Autodesk Inventor part; units mm, degrees
ref_plane "YZ Plane" through (0, 0, 0) normal (1, 0, 0) x (0, 1, 0)
ref_plane "XZ Plane" through (0, 0, 0) normal (0, 1, 0) x (-1, 0, 0)
ref_plane "XY Plane" through (0, 0, 0) normal (0, 0, 1) x (1, 0, 0)
sketch "Sketch1" plane through (0, 0, 0) normal (0, 1, 0) x (-1, 0, 0)
  line L0 (0, 0) -> (20, 0)
  line L1 (20, 0) -> (20, -20)
  line L2 (20, -20) -> (0, -20)
  line L3 (0, -20) -> (0, 0)
  point P0 (0, -10)
  point P1 (20, -10)
  dimension "d0" = 20
  dimension "d1" = 20
extrude "Extrusion1" add sketch "Sketch1" along normal blind 10
sketch "Sketch2" plane through (0, 0, 0) normal (0, -1, 0) x (1, 0, 0)
  circle A0 centre (-10, -10) radius 2.1511
  line L0 (-20, 0) -> (0, 0)
  line L1 (-13.8262, -12.1511) -> (-13.776, -7.7619)
  line L2 (-13.776, -7.7619) -> (-9.9498, -5.6108)
  line L3 (-9.9498, -5.6108) -> (-6.1738, -7.8489)
  line L4 (-6.1738, -7.8489) -> (-6.224, -12.2381)
  line L5 (-6.224, -12.2381) -> (-10.0502, -14.3892)
  line L6 (-10.0502, -14.3892) -> (-13.8262, -12.1511)
  dimension "d4" = 10
extrude "Extrusion2" cut sketch "Sketch2" against normal blind 1 contours A0 | L1 L2 L3 L4 L5 L6
sketch "Sketch3" plane through (0, 1, 0) normal (0, -1, 0) x (1, 0, 0)
  circle A0 centre (-9.9498, -10) radius 3
  line L0 (-20, 0) -> (0, 0)
  point P0 (-10, 0)
  dimension "d7" = 6
  dimension "d8" = 10
extrude "Extrusion3" cut sketch "Sketch3" against normal blind 8.5
sketch "Sketch4" plane through (0, 10, 0) normal (0, 1, 0) x (1, 0, 0)
  line L0 (0, 0) -> (0, 20)
  line L1 (-20, 20) -> (-20, 0)
  line L2 (0, 0) -> (-20, 20)
  line L3 (-20, 20) -> (-20, 0)
  line L4 (-20, 0) -> (0, 20)
  line L5 (0, 20) -> (0, 10)
  line L6 (0, 10) -> (-20, 10)
  line L7 (-20, 0) -> (0, 0)
  line L8 (-10, 0) -> (-10, 20)
  line L9 (-3.5295, 15.6) -> (-10, 15.6)
  line L10 (-10, 15.6) -> (-10, 12.6)
  line L11 (-10, 12.6) -> (-3.5295, 12.6)
  line L12 (-3.5295, 12.6) -> (-3.5295, 15.6)
  line L13 (-16.4705, 15.6) -> (-10, 15.6)
  line L14 (-10, 12.6) -> (-16.4705, 12.6)
  line L15 (-16.4705, 12.6) -> (-16.4705, 15.6)
  line L16 (-3.5295, 4.4) -> (-10, 4.4)
  line L17 (-10, 7.4) -> (-3.5295, 7.4)
  line L18 (-3.5295, 7.4) -> (-3.5295, 4.4)
  line L19 (-10, 7.4) -> (-16.4705, 7.4)
  line L20 (-16.4705, 7.4) -> (-16.4705, 4.4)
  line L21 (-16.4705, 4.4) -> (-10, 4.4)
  point P0 (-6.7648, 12.6)
  point P1 (-6.7648, 15.6)
  dimension "d11" = 3
  dimension "d18" = 5.2
extrude "Extrusion4" add sketch "Sketch4" along normal blind 10 contours L16 L8 L17 L2 | L2 L17 L18 L16 | L21 L4 L19 L8 | L9 L12 L11 L4 | L4 L11 L8 L9 | L14 L15 L13 L2 | L2 L13 L8 L14 | L4 L21 L20 L19
sketch "Sketch5" plane through (-3.5295, 10, -15.6) normal (0, 0, -1) x (-1, 0, 0)
  circle A0 centre (6.4705, 5) radius 2.75
  line L0 (0, 10) -> (12.941, 10)
  line L1 (16.4705, 0) -> (-3.5295, 0)
  line L2 (0, 0) -> (0, 10)
  line L3 (12.941, 0) -> (12.941, 10)
  point P0 (-3.5295, -10)
  dimension "d14" = 5.5
  dimension "d15" = 5
  dimension "d19" = 10
  dimension "d20" = 12.941
extrude "Extrusion5" cut sketch "Sketch5" against normal blind 66.5 contours A0
properties part number "RollZ" material "Thermoplastic Resin"
Geometry check sheet. Reference: the model listing, model coordinates, mm. A direction names the side the tool comes from. Coordinates: 2 decimals unless noted, no trailing zeros. Order: outer loops, then holes, each group sorted by start corner. A loop starts at its lowest first (then second) coordinate and runs counter-clockwise, first axis right, second up. Notation, with made-up numbers: (-19, -25.75) - (31, -25.75) arc R18 ccw to (31, -1.75) - close; hole circle Ø6 at (-21, 45). An arc over 180 degrees is marked (long way). Answer as a JSON object with one key per item and string values. Group by question number.
Item 1: Tool access check on faces 4 (the face through (-3.53, 15, -14)), 5 (the face through (-16.47, 15, -14)), 6 (the face through (-7, 15, -4.4)), 7 (the face through (-13, 15, -7.4)), 8 (the face through (-8.11, 0.49, -13.3)). Record the directions out of +Z, -Z, +X, -X, +Y, -Y that give a thin tool (end or side, any length) a straight path to the whole face; none if there is none.
Item 2: Depth check by flat-ended pin: pin 1 Ø3 at (x, y) = (-8.5, 15) entering from -Z; pin 2 Ø2.5 at (y, z) = (14, -13.5) entering from -X; pin 3 Ø1 at (x, z) = (-9.5, -3.5) entering from +Y. Enter the tip coordinate at first touch or a pass-through.
Item 3: Scan lines: probe 1 along Y at (x, z) = (-10, -14.9); probe 2 along Z at (x, y) = (-10.75, 18.25); probe 3 along Z at (x, y) = (-10, 6). Record each from-to range of solid material in increasing order.
Item 4: Sectioned sample at C-C, the plane y = 3.5. Record the cut outline in (x, z), and give its area (3 significant figures).
Item 5: Sectioned sample at A-A, the plane y = 15. Record the cut outline in (x, z), and give its area (3 significant figures).
Item 6: Sectioned sample at D-D, the plane x = -4.5. Record the cut outline in (y, z), and give its area (3 significant figures).
Item 7: Draft check along Z on faces 1 (the face through (-13, 15, -12.6)), 2 (the face through (-10, 5, -20)), 3 (the face through (-10, 20, -14)). Enter one of: +Z half, -Z half, draft (parallel to the pull), parting line (faces both ways), or undercut.
Item 8: Sectioned sample at B-B, the plane x = -8.25. Record the cut outline in (y, z).
Resolved:
{
 "1": {"face 4": "+Z, -Z, +X, +Y", "face 5": "+Z, -Z, -X, +Y", "face 6": "+Z, +X, -X, +Y", "face 7": "+X, -X, +Y", "face 8": "-Y"},
 "2": {"pin 1": "z = -15.6", "pin 2": "x = -16.47", "pin 3": "y = 10"},
 "3": {"probe 1": "0 to 12.25, 17.75 to 20", "probe 2": "-15.6 to -12.6, -7.4 to -4.4", "probe 3": "-20 to -13, -7 to 0"},
 "4": {"outline": "(-20, -20) - (0, -20) - (0, 0) - (-20, 0) - close; hole circle Ø6 at (-9.95, -10)", "area": "372 mm^2"},
 "5": {"outline": "(-16.47, -15.6) - (-12.75, -15.6) - (-12.75, -12.6) - (-16.47, -12.6) - close; (-16.47, -7.4) - (-12.75, -7.4) - (-12.75, -4.4) - (-16.47, -4.4) - close; (-7.25, -15.6) - (-3.53, -15.6) - (-3.53, -12.6) - (-7.25, -12.6) - close; (-7.25, -7.4) - (-3.53, -7.4) - (-3.53, -4.4) - (-7.25, -4.4) - close", "area": "44.6 mm^2"},
 "6": {"outline": "(0, -20) - (10, -20) - (10, -15.6) - (20, -15.6) - (20, -12.6) - (10, -12.6) - (10, -7.4) - (20, -7.4) - (20, -4.4) - (10, -4.4) - (10, 0) - (0, 0) - close", "area": "260 mm^2"},
 "7": {"face 1": "undercut", "face 2": "-Z half", "face 3": "draft"},
 "8": {"outline": "(0, -20) - (10, -20) - (10, -15.6) - (12.88, -15.6) - (12.88, -12.6) - (10, -12.6) - (10, -7.4) - (12.88, -7.4) - (12.88, -4.4) - (10, -4.4) - (10, 0) - (0, 0) - (0, -6.62) - (1, -6.62) - (1, -7.53) - (9.5, -7.53) - (9.5, -12.47) - (1, -12.47) - (1, -13.38) - (0, -13.38) - close; (17.12, -15.6) - (20, -15.6) - (20, -12.6) - (17.12, -12.6) - close; (17.12, -7.4) - (20, -7.4) - (20, -4.4) - (17.12, -4.4) - close"}
}
